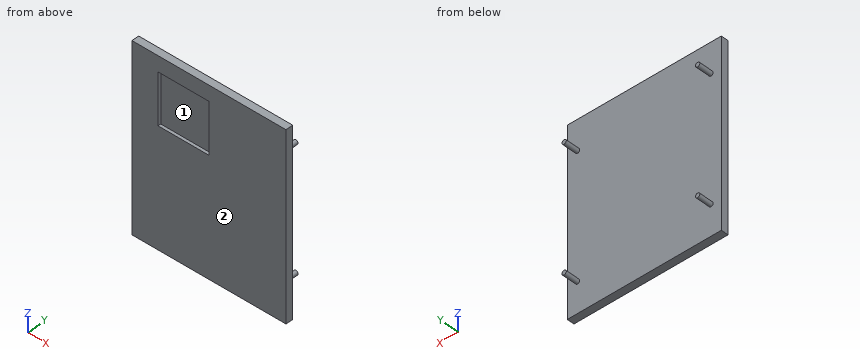
Autodesk Inventor part; units mm, degrees
ref_plane "YZ Plane" through (0, 0, 0) normal (1, 0, 0) x (0, 1, 0)
ref_plane "XZ Plane" through (0, 0, 0) normal (0, 1, 0) x (-1, 0, 0)
ref_plane "XY Plane" through (0, 0, 0) normal (0, 0, 1) x (1, 0, 0)
sketch "Boceto1" plane through (0, 0, 0) normal (0, 1, 0) x (-1, 0, 0)
  line L0 (53, 63) -> (-53, 63)
  line L1 (-53, 63) -> (-53, -63)
  line L2 (-53, -63) -> (53, -63)
  line L3 (53, -63) -> (53, 63)
  point P0 (0, 0)
  point P1 (0, 63)
  dimension "d1" = 106
  dimension "d2" = 126
  dimension "d3" = 53
  dimension "d4" = 63
extrude "Extrusión1" add sketch "Boceto1" along normal blind 5
sketch "Boceto2" plane through (0, 5, 0) normal (0, 1, 0) x (1, 0, 0)
  circle A0 centre (-45.929, -42.384) radius 1.5
  line L0 (-53, -63) -> (53, -63)
  line L1 (-53, 63) -> (-53, -63)
  line L2 (-81, 0) -> (77, 0)
  line L3 (0, -130) -> (0, 128)
  circle A1 centre (-45.929, 42.384) radius 1.5
  line L4 (-53, -63) -> (-53, 63)
  circle A2 centre (45.929, -42.384) radius 1.5
  circle A3 centre (45.929, 42.384) radius 1.5
  point P0 (0, 0)
  dimension "d7" = 3
  dimension "d8" = 20.616
  dimension "d9" = 7.071
extrude "Extrusión2" add sketch "Boceto2" along normal blind 10 contours A0 | A1 | A2 | A3
sketch "Boceto3" plane through (0, 0, 0) normal (0, -1, 0) x (1, 0, 0)
  line L0 (-35, 52.5) -> (35, 52.5)
  line L1 (35, 52.5) -> (35, -52.5)
  line L2 (35, -52.5) -> (-35, -52.5)
  line L3 (-35, -52.5) -> (-35, 52.5)
  line L4 (53, -63) -> (-53, -63)
  line L5 (-53, 63) -> (53, 63)
  line L6 (53, 63) -> (53, -63)
  line L7 (-53, -63) -> (-53, 63)
  line L8 (35, 17.5) -> (-35, 17.5)
  line L9 (35, -17.5) -> (-35, -17.5)
  line L10 (0, 52.5) -> (0, -52.5)
  point P0 (0, 0)
  point P1 (0, 17.5)
  dimension "d12" = 52.5
  dimension "d13" = 126
  dimension "d14" = 106
  dimension "d15" = 52.5
  dimension "d16" = 35
  dimension "d17" = 35
  dimension "d18" = 35
  dimension "d19" = 35
  dimension "d20" = 35
extrude "Extrusión3" cut sketch "Boceto3" against normal blind 2 contours L0 L10 L8 L3
properties part number "Tapa 0"
Verification items for the finished model (mm, model axes). Face numbers are marked on the shaded views. Give positions to 0.01 mm unless a question says otherwise; leave off trailing zeros. Loops run counter-clockwise (first coordinate to the right, second up) from the corner with the lowest first, then second, coordinate; pieces in that order, holes last.
1) Depth check by flat-ended pin: pin 1 Ø1.5 at (x, z) = (-37.5, 36) entering from +Y. Enter the tip coordinate at first touch or a pass-through.
2) Draft check along X on the marked faces 1 and 2. Enter one of: pulls with the +X half, pulls with the -X half, needs draft (parallel to the pull), parting line crosses it, or undercut.
3) Sectioned sample at D-D, the plane z = -39. Enter the section's corners in (x, y), then the cut area to 3 significant figures.
4) Sectioned sample at B-B, the plane x = -33.5. Enter the section's corners in (y, z).
5) Sectioned sample at A-A, the plane z = 23. Enter the section's corners in (x, y).
6) Sectioned sample at C-C, the plane y = 12. Enter the section's corners in (x, z), then the cut area to 3 significant figures.
7) Thickness scan on line 1 along X through (y, z) = (1, 26.5); line 2 along Z through (x, y) = (-21.5, 1); line 3 along Y through (x, z) = (-6.5, 6.5). Record the ranges inside material, lowest first.
Answers:
1. pin 1: stops at y = 5
2. face 1: undercut
2. face 2: needs draft
3. outline: (-53, 0) - (53, 0) - (53, 5) - (-53, 5) - close
3. area: 530 mm2
4. outline: (0, -63) - (5, -63) - (5, 63) - (0, 63) - (0, 52.5) - (2, 52.5) - (2, 17.5) - (0, 17.5) - close
5. outline: (-53, 0) - (-35, 0) - (-35, 2) - (0, 2) - (0, 0) - (53, 0) - (53, 5) - (-53, 5) - close
6. outline: circle Ø3 at (-45.93, -42.38); circle Ø3 at (-45.93, 42.38); circle Ø3 at (45.93, -42.38); circle Ø3 at (45.93, 42.38)
6. area: 28.3 mm2
7. line 1: x = -53 to -35, 0 to 53
7. line 2: z = -63 to 17.5, 52.5 to 63
7. line 3: y = 0 to 5
